```python
from build123d import *

# Parameters (mm, degrees)
SKETCH1_R           = 130
BOSS_EXTRUDE1_DEPTH = 10
CUT_EXTRUDE1_REACH  = 12
SKETCH2_R           = 35
SKETCH3_R           = 60
SKETCH3_R_2         = 50
BOSS_EXTRUDE2_DEPTH = 55
SKETCH4_R           = 130
SKETCH4_R_2         = 50
BOSS_EXTRUDE3_DEPTH = 5
SKETCH6_R           = 60
SKETCH6_R_2         = 45
BOSS_EXTRUDE4_DEPTH = 15
CUT_EXTRUDE3_DEPTH  = 5
CIRPATTERN1_COUNT   = 7
SKETCH10_R          = 115
SKETCH10_R_2        = 112
BOSS_EXTRUDE5_DEPTH = 15
SKETCH11_W          = 5
SKETCH11_H          = 25
CUT_EXTRUDE4_DEPTH  = 15
CIRPATTERN2_COUNT   = 7
SKETCH12_R          = 10
CUT_EXTRUDE5_DEPTH  = 10
CIRPATTERN3_COUNT   = 7
FILLET1_R           = 5


with BuildPart() as part:
    # Sketch1 → Boss-Extrude1 (new body)
    with BuildSketch(Plane(origin=(0, 0, 0), x_dir=(1, 0, 0), z_dir=(0, 1, 0))):
        Circle(SKETCH1_R)
    extrude(amount=BOSS_EXTRUDE1_DEPTH)

    # Sketch2 → Cut-Extrude1 (cut, up to next)
    with BuildSketch(Plane(origin=(0, 10, 0), x_dir=(1, 0, 0), z_dir=(0, 1, 0)), mode=Mode.PRIVATE) as cut_extrude1_sk1:
        Circle(SKETCH2_R)
    cut_extrude1_tool1 = extrude(cut_extrude1_sk1.sketch, amount=-CUT_EXTRUDE1_REACH, mode=Mode.PRIVATE) & part.part
    add(cut_extrude1_tool1.solids().sort_by_distance((0, 10, 0))[0], mode=Mode.SUBTRACT)

    # Sketch3 → Boss-Extrude2 (add)
    with BuildSketch(Plane(origin=(0, 10, 0), x_dir=(1, 0, 0), z_dir=(0, 1, 0))):
        Circle(SKETCH3_R)
        Circle(SKETCH3_R_2, mode=Mode.SUBTRACT)
    extrude(amount=BOSS_EXTRUDE2_DEPTH)

    # Sketch4 → Boss-Extrude3 (add)
    with BuildSketch(Plane(origin=(0, 65, 0), x_dir=(1, 0, 0), z_dir=(0, 1, 0))):
        Circle(SKETCH4_R)
        Circle(SKETCH4_R_2, mode=Mode.SUBTRACT)
    extrude(amount=BOSS_EXTRUDE3_DEPTH)

    # Sketch6 → Boss-Extrude4 (add)
    with BuildSketch(Plane.XZ):
        Circle(SKETCH6_R)
        Circle(SKETCH6_R_2, mode=Mode.SUBTRACT)
    extrude(amount=BOSS_EXTRUDE4_DEPTH)

    # Sketch8 → Cut-Extrude3 (cut)
    with BuildSketch(Plane(origin=(0, 70, 0), x_dir=(1, 0, 0), z_dir=(0, 1, 0))):
        with BuildLine():
            Line((40, -110), (40, -123.693168769))
            ThreePointArc((40, -123.693168769), (0, -130), (-40, -123.693168769))
            Line((-40, -123.693168769), (-40, -110))
            ThreePointArc((-40, -110), (0, -70), (40, -110))
        make_face()
    cut_extrude3 = extrude(amount=-CUT_EXTRUDE3_DEPTH, mode=Mode.SUBTRACT)

    # CirPattern1: Cut-Extrude3 ×7 about axis
    cirpattern1_axis = Axis((0, 0, 0), (0, 1, 0))
    for i in range(1, CIRPATTERN1_COUNT):
        add(cut_extrude3.rotate(cirpattern1_axis, i * 360 / CIRPATTERN1_COUNT), mode=Mode.SUBTRACT)

    # Sketch10 → Boss-Extrude5 (add)
    with BuildSketch(Plane.XZ):
        Circle(SKETCH10_R)
        Circle(SKETCH10_R_2, mode=Mode.SUBTRACT)
    extrude(amount=BOSS_EXTRUDE5_DEPTH)

    # Sketch11 → Cut-Extrude4 (cut)
    with BuildSketch(Plane.XZ.offset(15)):
        with Locations((0, 110)):
            Rectangle(SKETCH11_W, SKETCH11_H)
    cut_extrude4 = extrude(amount=-CUT_EXTRUDE4_DEPTH, mode=Mode.SUBTRACT)

    # CirPattern2: Cut-Extrude4 ×7 about axis
    cirpattern2_axis = Axis((0, 0, 0), (0, 1, 0))
    for i in range(1, CIRPATTERN2_COUNT):
        add(cut_extrude4.rotate(cirpattern2_axis, i * 360 / CIRPATTERN2_COUNT), mode=Mode.SUBTRACT)

    # Sketch12 → Cut-Extrude5 (cut)
    with BuildSketch(Plane(origin=(0, 10, 0), x_dir=(1, 0, 0), z_dir=(0, 1, 0))):
        with Locations((0, -100)):
            Circle(SKETCH12_R)
    cut_extrude5 = extrude(amount=-CUT_EXTRUDE5_DEPTH, mode=Mode.SUBTRACT)

    # CirPattern3: Cut-Extrude5 ×7 about axis
    cirpattern3_axis = Axis((0, 0, 0), (0, 1, 0))
    for i in range(1, CIRPATTERN3_COUNT):
        add(cut_extrude5.rotate(cirpattern3_axis, i * 360 / CIRPATTERN3_COUNT), mode=Mode.SUBTRACT)

    # Fillet1
    fillet1_edges = [part.edges().sort_by_distance(p)[0] for p in [
        (71.767621435, 67.5, 108.394688585),
        (121.646805584, 67.5, 45.848169988),
        (-40, 67.5, 123.693168769),
        (40, 67.5, 123.693168769),
        (-121.646805584, 67.5, 45.848169988),
        (-71.767621435, 67.5, 108.394688585),
        (-17.629699852, 67.5, -128.799043797),
        (-89.707209285, 67.5, -94.088344668),
        (-111.69108542, 67.5, -66.521435926),
        (-129.492760137, 67.5, 11.472797049),
        (129.492760137, 67.5, 11.472797049),
        (111.69108542, 67.5, -66.521435926),
        (89.707209285, 67.5, -94.088344668),
        (17.629699852, 67.5, -128.799043797),
    ]]
    fillet(fillet1_edges, radius=FILLET1_R)


solid = part.part
```
Work out the finished part from the listing and answer in its coordinate system (mm). A direction names the side the tool comes from. Round coordinates to 2 decimals unless told otherwise and drop trailing zeros. Write each loop counter-clockwise with the first axis right and the second up, starting at its lowest first coordinate (ties: lowest second). Pieces come first, ordered by that corner, then holes.
1) Flat-ended cylindrical pins translate along their axes: P1, Ø2, axis at y = 11.5, z = -30.5, coming from the +X side; P2, Ø4, axis at x = -23, y = -6, coming from the +Z side; P3, Ø5, axis at x = 4.5, y = 51.5, coming from the +Z side; P4, Ø12, axis at x = -97.49, z = -22.25, coming from the +Y side. Find the tip coordinate at first contact, or state that the pin passes through.
2) A cutting plane is placed at B-B on y = 41.5. Determine the outline of the cut face in (x, z).
3) Consider probe 1 along Z at (x, y) = (0, 5); probe 2 along Y at (x, z) = (-94, -84.5); probe 3 along X at (y, z) = (-10.5, 46). Determine where each line is inside the solid, lowest interval first.
4) Which of the six approach directions +Z, -Z, +X, -X, +Y, -Y give full straight-line access (tool end or side, diameter ignored) to faces 1 (the face through (-59.94, -7.4, 2.64)), 2 (the face through (-29.58, 67.54, -63.46)), 3 (the face through (-0.688, -7.395, -114.998)), 4 (the face through (-1, 65, -61))?
5) A cutting plane is placed at A-A on z = 95. Determine the outline of the cut face in (x, y).
6) Determine the mould class of faces 5 (the face through (-0.88, 67.54, 70.01)), 6 (the face through (-109.041, -7.395, 25.574)), 7 (the face through (-49.276, -7.395, 103.908)), 8 (the face through (9, -15, 45)) for opening direction X: pulls with the +X half, pulls with the -X half, needs draft (parallel to the pull), parting line crosses it, or undercut.
Entries:
1. P1: stops at x = 52.25
1. P2: stops at z = 113.07
1. P3: stops at z = 59.97
1. P4: passes through
2. outline: circle Ø120 at (0, 0); hole circle Ø100 at (0, 0)
3. probe 1: z = -130 to -35, 35 to 90, 110 to 130
3. probe 2: y = 0 to 10, 65 to 70
3. probe 3: x = -105.4 to -102.12, -38.52 to 38.52, 102.12 to 105.4
4. face 1: -Y
4. face 2: +Y
4. face 3: -Z, -Y
4. face 4: none
5. outline: (-88.74, 0) - (-64.81, 0) - (-64.81, -15) - (-59.32, -15) - (-59.32, 0) - (-8.66, 0) - (-8.66, 10) - (-88.74, 10) - close; (-55.97, 65) - (-37.08, 65) - (-37.08, 70) - (-55.97, 70) - close; (8.66, 0) - (59.32, 0) - (59.32, -15) - (64.81, -15) - (64.81, 0) - (88.74, 0) - (88.74, 10) - (8.66, 10) - close; (37.08, 65) - (55.97, 65) - (55.97, 70) - (37.08, 70) - close
6. face 5: undercut
6. face 6: undercut
6. face 7: pulls with the -X half
6. face 8: needs draft
